Geometry check sheet. Reference: the model listing, model coordinates, mm. A direction names the side the tool comes from. Coordinates: 2 decimals unless noted, no trailing zeros. Write each loop counter-clockwise with the first axis right and the second up, starting at its lowest first coordinate (ties: lowest second). Pieces come first, ordered by that corner, then holes. Notation, with made-up numbers: (-22.5, 7.25) -> (34.5, 7.25) arc R20 cw to (34.5, 13.25) -> close; hole circle Ø4 at (-0.5, 50). An arc over 180 degrees is marked (long way). Answer in a Markdown table with one row per item. Add a question column.
1. Scan lines: L1, parallel to Y at x = -15.5, z = -28.45; L2, parallel to Y at x = 0, z = -27; L3, parallel to Y at x = -15.5, z = -32. Record each from-to range of solid material in increasing order. Write a range as from..to.
2. Set-up check for faces 1 (the flat face through (14, 14, -30)), 2 (the flat face through (-19, 57.25, -30)), 3 (the flat face through (27.5, 23, -11)): record each of +Z, -Z, +X, -X, +Y, -Y from which the full face is reachable in a straight line by a thin tool's end or side.
3. Mould release check, pull along Z, two halves, no side actions. Record for faces 4 (the flat face through (-27.5, 23, -11)), 5 (the flat face through (7, 42, -35)), 6 (the cylindrical face through (-17.29, 64.45, -28.34)): pulls with the +Z half, pulls with the -Z half, needs draft (parallel to the pull), parting line crosses it, or undercut.
4. Cross-section at A-A on x = 0. Record the cut outline in (y, z).
5. Cross-section at B-B on y = 61.5. Record the cut outline in (x, z), and give its area (3 significant figures).
6. Cross-section at D-D on y = 15.65. Record the cut outline in (x, z), and give its area (3 significant figures).
7. Depth check by flat-ended pin: P1, Ø8, axis at x = -24.5, z = -15, coming from the -Y side; P2, Ø1.5, axis at x = 24, z = -13.5, coming from the +Y side; P3, Ø6, axis at x = -15.5, y = 21, coming from the +Z side; P4, Ø3, axis at x = 15, y = 14.5, coming from the -Z side. Enter the tip coordinate at first touch or a pass-through.
8. Cross-section at C-C on x = 8. Record the cut outline in (y, z), and give its area (3 significant figures).
```python
from build123d import *

# Parameters (mm, degrees)
SKETCH1_W           = 65
SKETCH1_H           = 70
BOSS_EXTRUDE1_DEPTH = 10
SKETCH2_W           = 65
SKETCH2_H           = 10
BOSS_EXTRUDE2_DEPTH = 60
FILLET1_R           = 10
CUT_EXTRUDE3_DEPTH  = 60
FILLET2_R           = 10
FILLET3_R           = 1
FILLET4_R           = 1
SKETCH4_R           = 11.1
CUT_EXTRUDE4_DEPTH  = 60
RIB1_REACH          = 103.735
SKETCH5_WALL_W      = 265.86260353
SKETCH5_WALL_H      = 5
SKETCH6_R           = 1.8
CUT_EXTRUDE5_DEPTH  = 20
SKETCH7_R           = 1.8
CUT_EXTRUDE8_DEPTH  = 10
SKETCH9_R           = 3
CUT_EXTRUDE9_DEPTH  = 5


with BuildPart() as part:
    # Sketch1 → Boss-Extrude1 (new body)
    with BuildSketch(Plane(origin=(0, 0, 0), x_dir=(1, 0, 0), z_dir=(0, 1, 0))):
        Rectangle(SKETCH1_W, SKETCH1_H)
    extrude(amount=BOSS_EXTRUDE1_DEPTH)

    # Sketch2 → Boss-Extrude2 (add)
    with BuildSketch(Plane(origin=(0, 10, 0), x_dir=(1, 0, 0), z_dir=(0, 1, 0))):
        with Locations((0, 30)):
            Rectangle(SKETCH2_W, SKETCH2_H)
    extrude(amount=BOSS_EXTRUDE2_DEPTH)

    # Fillet1
    fillet1_edges = [part.edges().sort_by_distance(p)[0] for p in [
        (-32.5, 5, 35),
        (32.5, 5, 35),
    ]]
    fillet(fillet1_edges, radius=FILLET1_R)

    # Sketch3 → Cut-Extrude3 (cut)
    with BuildSketch(Plane.XY.offset(-25)):
        with BuildLine():
            Line((-5.95294045, 58.75), (-32.5, 58.75))
            Line((-32.5, 58.75), (-32.5, 57.25))
            Line((-32.5, 57.25), (-5.95294045, 57.25))
            ThreePointArc((-5.95294045, 57.25), (6, 58), (-5.95294045, 58.75))
        make_face()
    extrude(amount=-CUT_EXTRUDE3_DEPTH, mode=Mode.SUBTRACT)

    # Fillet2
    fillet2_edges = [part.edges().sort_by_distance(p)[0] for p in [
        (-32.5, 70, -30),
        (32.5, 70, -30),
    ]]
    fillet(fillet2_edges, radius=FILLET2_R)

    # Fillet3
    fillet3_edges = [part.edges().sort_by_distance(p)[0] for p in [
        (-32.5, 58.75, -30),
    ]]
    fillet(fillet3_edges, radius=FILLET3_R)

    # Fillet4
    fillet4_edges = [part.edges().sort_by_distance(p)[0] for p in [
        (-32.5, 57.25, -30),
    ]]
    fillet(fillet4_edges, radius=FILLET4_R)

    # Sketch4 → Cut-Extrude4 (cut)
    with BuildSketch(Plane.XY.offset(-25)):
        with Locations((0, 31.15)):
            Circle(SKETCH4_R)
    extrude(amount=-CUT_EXTRUDE4_DEPTH, mode=Mode.SUBTRACT)

    # Sketch5 wall → Rib1 (add, up to next)
    with BuildSketch(Plane(origin=(-32.5, 30.832944907, -3.141178401), x_dir=(0, -0.689915950612, 0.723889481269), z_dir=(0, 0.723889481269, 0.689915950612)), mode=Mode.PRIVATE) as rib1_sk1:
        with Locations((0, 2.5)):
            Rectangle(SKETCH5_WALL_W, SKETCH5_WALL_H)
    rib1_tool1 = extrude(rib1_sk1.sketch, amount=-RIB1_REACH, mode=Mode.PRIVATE) - part.part
    rib1 = rib1_tool1.solids().sort_by_distance((-32.5, 30.832944907, -3.141178401))[0]
    add(rib1)

    # Mirror1: Rib1 across plane
    add(rib1.mirror(Plane(origin=(0, 0, 0), x_dir=(0, 0, 1), z_dir=(1, 0, 0))))

    # Sketch6 → Cut-Extrude5 (cut)
    with BuildSketch(Plane(origin=(0, 70, 0), x_dir=(1, 0, 0), z_dir=(0, 1, 0))):
        with Locations(Location((-16.597294225, 30, 0), (0, 0, 270))):
            Circle(SKETCH6_R)
    extrude(amount=-CUT_EXTRUDE5_DEPTH, mode=Mode.SUBTRACT)

    # Sketch7 → Cut-Extrude8 (cut)
    with BuildSketch(Plane.XY.offset(-25)):
        with Locations((-15.5, 46.65)):
            Circle(SKETCH7_R)
        with Locations((15.5, 46.65)):
            Circle(SKETCH7_R)
        with Locations((15.5, 15.65)):
            Circle(SKETCH7_R)
        with Locations((-15.5, 15.65)):
            Circle(SKETCH7_R)
    extrude(amount=-CUT_EXTRUDE8_DEPTH, mode=Mode.SUBTRACT)

    # Sketch9 → Cut-Extrude9 (cut)
    with BuildSketch(Plane(origin=(0, 0, -35), x_dir=(-1, 0, 0), z_dir=(0, 0, -1))):
        with Locations((-15.5, 46.65)):
            Circle(SKETCH9_R)
        with Locations((15.5, 46.65)):
            Circle(SKETCH9_R)
        with Locations((15.5, 15.65)):
            Circle(SKETCH9_R)
        with Locations((-15.5, 15.65)):
            Circle(SKETCH9_R)
    extrude(amount=-CUT_EXTRUDE9_DEPTH, mode=Mode.SUBTRACT)


solid = part.part
```
Results found:
| question | item | result |
|---|---|---|
| 1 | L1 | y = 0..13.85, 17.45..44.85, 48.45..57.25, 58.75..70 |
| 1 | L2 | y = 0..20.05, 42.25..52, 64..70 |
| 1 | L3 | y = 0..12.65, 18.65..43.65, 49.65..57.25, 58.75..70 |
| 2 | face 1 | -Z |
| 2 | face 2 | +Z, -Z, -X |
| 2 | face 3 | +Z, +Y |
| 3 | face 4 | needs draft |
| 3 | face 5 | pulls with the -Z half |
| 3 | face 6 | undercut |
| 4 | outline | (0, -35) -> (20.05, -35) -> (20.05, -25) -> (10, -25) -> (10, 35) -> (0, 35) -> close; (42.25, -35) -> (52, -35) -> (52, -25) -> (42.25, -25) -> close; (64, -35) -> (70, -35) -> (70, -25) -> (64, -25) -> close |
| 5 | outline | (-32.39, -35) -> (-4.87, -35) -> (-4.87, -25) -> (-32.39, -25) -> close; (4.87, -35) -> (32.39, -35) -> (32.39, -25) -> (4.87, -25) -> close; hole circle Ø3.6 at (-16.6, -30) |
| 5 | area | 540 mm^2 |
| 6 | outline | (-32.5, -35) -> (-18.5, -35) -> (-18.5, -30) -> (-17.3, -30) -> (-17.3, -25) -> (-27.5, -25) -> (-27.5, 12.79) -> (-32.5, 12.79) -> close; (-13.7, -30) -> (-12.5, -30) -> (-12.5, -35) -> (12.5, -35) -> (12.5, -30) -> (13.7, -30) -> (13.7, -25) -> (-13.7, -25) -> close; (17.3, -30) -> (18.5, -30) -> (18.5, -35) -> (32.5, -35) -> (32.5, 12.79) -> (27.5, 12.79) -> (27.5, -25) -> (17.3, -25) -> close |
| 6 | area | 932 mm^2 |
| 7 | P1 | stops at y = 0 |
| 7 | P2 | stops at y = 10 |
| 7 | P3 | stops at z = -25 |
| 7 | P4 | stops at z = -30 |
| 8 | outline | (0, -35) -> (23.46, -35) -> (23.46, -25) -> (10, -25) -> (10, 35) -> (0, 35) -> close; (38.84, -35) -> (70, -35) -> (70, -25) -> (38.84, -25) -> close |
| 8 | area | 1,150 mm^2 |
